from build123d import *

# Parameters (mm, degrees)
CHAMFER1_SIZE      = 0.25
FILLET1_R          = 0.2
CUT_EXTRUDE1_DEPTH = 1.25
FILLET2_R          = 0.1


with BuildPart() as part:
    # Sketch1 → Revolve1 (revolve)
    with BuildSketch(Plane.XY, mode=Mode.PRIVATE) as revolve1_sk:
        Polygon((0, -18.5), (-1.25, -18.5), (-1.25, -2.5), (-2.25, -2.5), (-2.25, 0), (0, 0), align=None)
    revolve(revolve1_sk.sketch.rotate(Axis((0, 0, 0), (0, -1, 0)), 270), axis=Axis((0, 0, 0), (0, -1, 0)))

    # Chamfer1
    chamfer1_edges = [part.edges().sort_by_distance(p)[0] for p in [
        (0, -2.5, -1.25),
        (0, -18.5, -1.25),
    ]]
    chamfer(chamfer1_edges, length=CHAMFER1_SIZE)

    # Fillet1
    fillet1_edges = [part.edges().sort_by_distance(p)[0] for p in [
        (0, 0, -2.25),
    ]]
    fillet(fillet1_edges, radius=FILLET1_R)

    # Sketch2 → Cut-Extrude1 (cut)
    with BuildSketch(Plane(origin=(0, 0, 0), x_dir=(1, 0, 0), z_dir=(0, 1, 0))):
        Polygon((0, 1.154700538), (-1, 0.577350269), (-1, -0.577350269), (0, -1.154700538), (1, -0.577350269), (1, 0.577350269), align=None)
    extrude(amount=-CUT_EXTRUDE1_DEPTH, mode=Mode.SUBTRACT)

    # Fillet2
    fillet2_edges = [part.edges().sort_by_distance(p)[0] for p in [
        (0.5, -1.25, -0.866025404),
        (1, -1.25, 0),
        (0.5, -1.25, 0.866025404),
        (-0.5, -1.25, 0.866025404),
        (-1, -1.25, 0),
        (-0.5, -1.25, -0.866025404),
        (0.4999999999999987, 0, -0.8660254037844397),
        (-0.5000000000000006, 0, -0.8660254037844395),
        (-1, 0, 0),
        (-0.5000000000000007, 0, 0.8660254037844379),
        (0.4999999999999988, 0, 0.8660254037844382),
        (1, 0, 0),
    ]]
    fillet(fillet2_edges, radius=FILLET2_R)


solid = part.part
CAD build for the part. Positions are in the model's coordinates, mm. A direction names the side the tool comes from. Round coordinates to 2 decimals unless told otherwise and drop trailing zeros. Loops run counter-clockwise (first coordinate to the right, second up) from the corner with the lowest first, then second, coordinate; pieces in that order, holes last.
(1) Cut at A-A (z = 0). Give the cut face in (x, y), plus the area to 3 significant figures.
(2) Wall check: line 1 along Y through (x, z) = (-1.25, 0.85); line 2 along Y through (x, z) = (0.55, -0.5); line 3 along X through (y, z) = (-3.5, -0.25). Give the ranges that are in metal, low to high.
(3) Cut at B-B (y = -4.5). Give the cut face in (x, z).
(4) Which spindle directions (+Z, -Z, +X, -X, +Y, -Y) get a long thin tool onto all of the face, cutting with end or side? Do faces 4 (the flat face through (0, -18.5, 0)), 5 (the flat face through (0, -1.25, 0)), 6 (the cylindrical face through (1.22, -10.39, -0.27)). Say none if no direction does.
(5) Two-plate mould, pull along Z, no slides. Class faces 1 (the flat face through (-0.49, -0.62, -0.87)), 2 (the flat face through (0, -2.5, 2)), 3 (the cylindrical face through (-0.676, -1.334, 2.146)): +Z half, -Z half, draft (parallel to the pull), parting line (faces both ways), or undercut.
(6) Drop a flat-ended pin along its axis: pin 1 (0.5 mm diameter, centred on x = 0, z = 0, fed in from +Y). Give the stop position or say it passes through.
Findings below:
1. outline: (-2.25, -2.5) - (-1.5, -2.5) - (-1.25, -2.75) - (-1.25, -18.25) - (-1, -18.5) - (1, -18.5) - (1.25, -18.25) - (1.25, -2.75) - (1.5, -2.5) - (2.25, -2.5) - (2.25, -0.2) arc R0.2 ccw to (2.05, 0) - (1.1, 0) arc R0.1 ccw to (1, -0.1) - (1, -1.15) arc R0.1 cw to (0.9, -1.25) - (-0.9, -1.25) arc R0.1 cw to (-1, -1.15) - (-1, -0.1) arc R0.1 ccw to (-1.1, 0) - (-2.05, 0) arc R0.2 ccw to (-2.25, -0.2) - close
1. area: 48.7 mm2
2. line 1: y = -2.5 to 0
2. line 2: y = -18.5 to -1.25
2. line 3: x = -1.22 to 1.22
3. outline: circle Ø2.5 at (0, 0)
4. face 4: +Z, -Z, +X, -X, -Y
4. face 5: +Y
4. face 6: -Y
5. face 1: undercut
5. face 2: draft
5. face 3: parting line
6. pin 1: stops at y = -1.25
